Check sheet for the drawn part. Datum: minimum x, y, z corner. Units: mm. Coordinates: 2 decimals unless noted, no trailing zeros. Order: outer loops, then holes, each group sorted by start corner. A loop starts at its lowest first (then second) coordinate and runs counter-clockwise, first axis right, second up. Notation, with made-up numbers: (68.5, -13.5) - (127.5, -13.5) arc R6 ccw to (127.5, -7.5) - close; hole circle Ø3 at (-5.75, -36.5). An arc over 180 degrees is marked (long way). One line per item, written item: value. Start each with the question number.
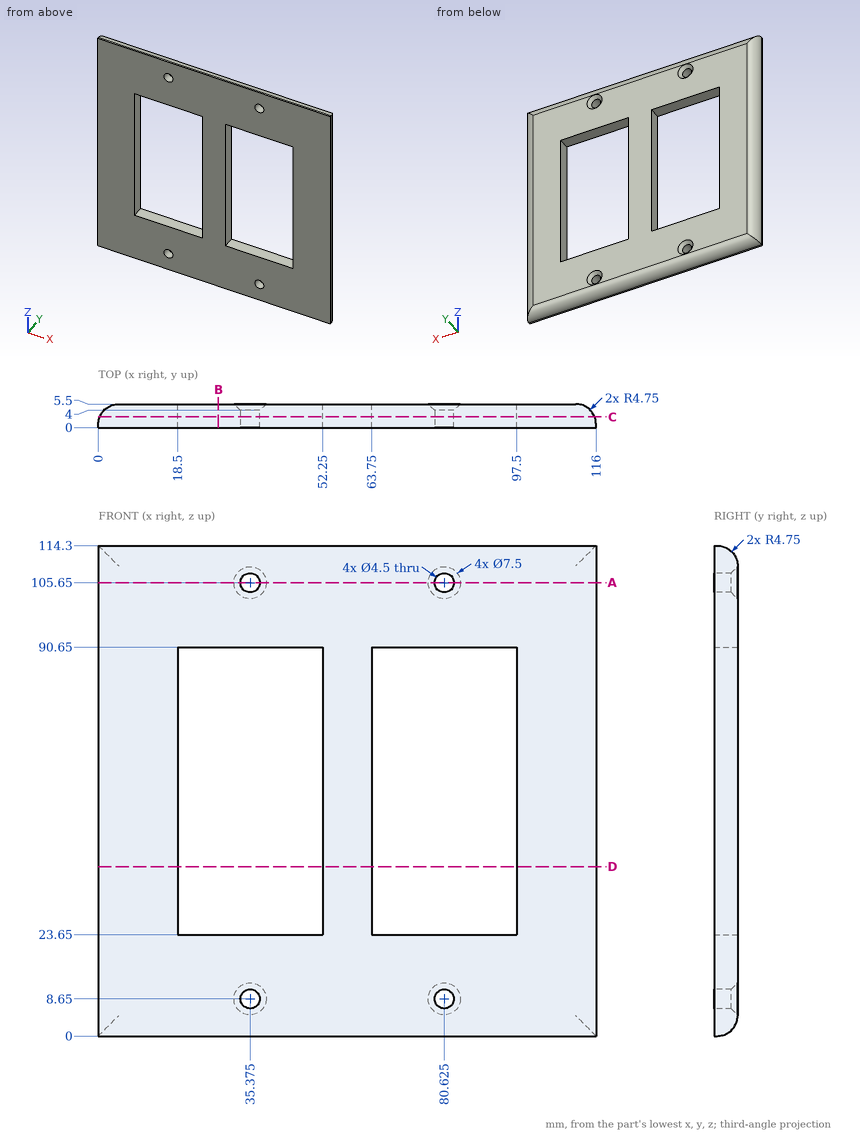
Q1. Material ranges on probe 1 along Z at (x, y) = (79.5, 3.65); probe 2 along X at (y, z) = (3.3, 87); probe 3 along X at (y, z) = (4.7, 105), recorded low to high.
Q2. Cross-section at D-D, the plane z = 39.5. Enter the section's corners in (x, y).
Q3. Gauge pin test, flat ends, axial feed: P1, Ø3, axis at x = 31.5, y = 3, coming from the -Z side; P2, Ø2, axis at x = 24.5, y = 2.5, coming from the +Z side; P3, Ø1.6, axis at x = 84.5, y = 2, coming from the -Z side. Record the tip position at first contact, or that the pin passes through.
Q4. Cross-section at C-C, the plane y = 2.5. Enter the section's corners in (x, z) (3 decimals).
Q5. Cross-section at B-B, the plane x = 28. Enter the section's corners in (y, z), and give its area (3 significant figures).
Q6. Cross-section at A-A, the plane z = 105.65. Enter the section's corners in (x, y) (3 decimals).
Check result:
1. probe 1: z = 0.99 to 6.7, 10.6 to 23.65, 90.65 to 103.7, 107.6 to 113.31
1. probe 2: x = 0.74 to 18.5, 52.25 to 63.75, 97.5 to 115.26
1. probe 3: x = 2.11 to 32.5, 38.25 to 77.75, 83.5 to 113.89
2. outline: (0, 0) - (18.5, 0) - (18.5, 5.5) - (4.75, 5.5) arc R4.75 ccw to (0, 0.75) - close; (52.25, 0) - (63.75, 0) - (63.75, 5.5) - (52.25, 5.5) - close; (97.5, 0) - (116, 0) - (116, 0.75) arc R4.75 ccw to (111.25, 5.5) - (97.5, 5.5) - close
3. P1: stops at z = 0.06
3. P2: stops at z = 114.24
3. P3: stops at z = 0.02
4. outline: (0.334, 0.334) - (115.666, 0.334) - (115.666, 113.966) - (0.334, 113.966) - close; hole (18.5, 23.65) - (52.25, 23.65) - (52.25, 90.65) - (18.5, 90.65) - close; hole circle Ø4.5 at (35.375, 8.65); hole circle Ø4.5 at (35.375, 105.65); hole (63.75, 23.65) - (97.5, 23.65) - (97.5, 90.65) - (63.75, 90.65) - close; hole circle Ø4.5 at (80.625, 8.65); hole circle Ø4.5 at (80.625, 105.65)
5. outline: (0, 0) - (0.75, 0) arc R4.75 ccw to (5.5, 4.75) - (5.5, 23.65) - (0, 23.65) - close; (0, 90.65) - (5.5, 90.65) - (5.5, 109.55) arc R4.75 ccw to (0.75, 114.3) - (0, 114.3) - close
5. area: 250 mm2
6. outline: (0, 0) - (33.125, 0) - (33.125, 4) - (31.625, 5.5) - (4.75, 5.5) arc R4.75 ccw to (0, 0.75) - close; (37.625, 0) - (78.375, 0) - (78.375, 4) - (76.875, 5.5) - (39.125, 5.5) - (37.625, 4) - close; (82.875, 0) - (116, 0) - (116, 0.75) arc R4.75 ccw to (111.25, 5.5) - (84.375, 5.5) - (82.875, 4) - close
